from build123d import *

# Parameters (mm, degrees)
SKETCH1_W                        = 25.4
SKETCH1_H                        = 50.8
SKETCH1_W_2                      = 19.05
SKETCH1_H_2                      = 44.45
EXTRUDE_THIN1_DEPTH              = 571.5
F_8_CLEARANCE_HOLE1_D            = 4.4958
F_1_8_0_135_DIAMETER_HOLE1_D     = 3.429
F_1_8_0_135_DIAMETER_HOLE1_DEPTH = 3.175


with BuildPart() as part:
    # Sketch1 → Extrude-Thin1 (new body)
    with BuildSketch(Plane.XY):
        Rectangle(SKETCH1_W, SKETCH1_H)
        Rectangle(SKETCH1_W_2, SKETCH1_H_2, mode=Mode.SUBTRACT)
    extrude(amount=EXTRUDE_THIN1_DEPTH)

    # #8 Clearance Hole1 (through all)
    with Locations(Plane(origin=(0, 25.4, 565.15), x_dir=(0, 0, 1), z_dir=(0, 1, 0))):
        with Locations((0, 0), (-558.8, 0), (-533.4, 0), (-508, 0), (-25.4, 0), (-50.8, 0)):
            Hole(F_8_CLEARANCE_HOLE1_D / 2)

    # 1/8 (0.135) Diameter Hole1
    with Locations(Plane(origin=(0, 25.4, 0), x_dir=(1, 0, 0), z_dir=(0, 1, 0))):
        with Locations((-3.175, -82.555663772), (3.175, -107.955663772), (-3.175, -133.355663772), (3.175, -158.755663772), (-3.175, -184.155663772), (3.175, -209.555663772), (-3.175, -234.955663772), (3.175, -260.355663772), (-3.175, -285.755663772), (3.175, -311.155663772), (-3.175, -336.555663772), (3.175, -361.955663772), (-3.175, -387.355663772), (3.175, -412.755663772), (-3.175, -438.155663772), (3.175, -463.555663772), (-3.175, -488.955663772)):
            Hole(F_1_8_0_135_DIAMETER_HOLE1_D / 2, depth=F_1_8_0_135_DIAMETER_HOLE1_DEPTH)


solid = part.part
Check sheet for the modelled part. Datum: model origin and axes. Units: mm. A direction names the side the tool comes from. Coordinates: 2 decimals unless noted, no trailing zeros. Write each loop counter-clockwise with the first axis right and the second up, starting at its lowest first coordinate (ties: lowest second). Pieces come first, ordered by that corner, then holes.
Item 1: Mould release check, pull along X, two halves, no side actions. Record for faces 1 (the face through (12.7, 0, 282)), 2 (the face through (0, 22.225, 282)), 3 (the face through (0, -25.4, 282)), 4 (the face through (-9.525, 0, 282)): released by +X, released by -X, zero draft, split by the parting line, or undercut.
Numbers:
face 1: released by +X
face 2: undercut
face 3: zero draft
face 4: undercut
Item 2: Depth check by flat-ended pin: pin 1 Ø3 at (x, z) = (3.18, 107.96) entering from +Y (3 decimals); pin 2 Ø4 at (x, z) = (0, 539.75) entering from +Y. Enter the tip coordinate at first touch or a pass-through.
Numbers:
pin 1: stops at y = -22.225
pin 2: passes through
Item 3: Cross-section at A-A on z = 126. Record the boundary of the cut face in (x, y) (3 decimals), then the cut area to 3 significant figures.
Numbers:
outline: (-12.7, -25.4) - (12.7, -25.4) - (12.7, 25.4) - (-12.7, 25.4) - close; hole (-9.525, -22.225) - (9.525, -22.225) - (9.525, 22.225) - (-9.525, 22.225) - close
area: 444 mm2
Item 4: Access from +Z, -Z, +X, -X, +Y, -Y to the whole of each face (thin tool, end or side, straight path). Record for faces 5 (the face through (9.525, 0, 282)), 6 (the face through (-10, -2, 0)).
Numbers:
face 5: +Z, -Z
face 6: -Z, +X, -X, +Y, -Y
Item 5: Scan lines: probe 1 along X at (y, z) = (-24, 57); probe 2 along X at (y, z) = (-3, 369.5) (3 decimals); probe 3 along Y at (x, z) = (-7.5, 157.5) (3 decimals). Record each from-to range of solid material in increasing order.
Numbers:
probe 1: x = -12.7 to -2.24, 2.24 to 12.7
probe 2: x = -12.7 to -9.525, 9.525 to 12.7
probe 3: y = -25.4 to -22.225, 22.225 to 25.4
Item 6: Cross-section at B-B on y = 6.5. Record the boundary of the cut face in (x, z) (3 decimals), then the cut area to 3 significant figures.
Numbers:
outline: (-12.7, 0) - (-9.525, 0) - (-9.525, 571.5) - (-12.7, 571.5) - close; (9.525, 0) - (12.7, 0) - (12.7, 571.5) - (9.525, 571.5) - close
area: 3,630 mm2
